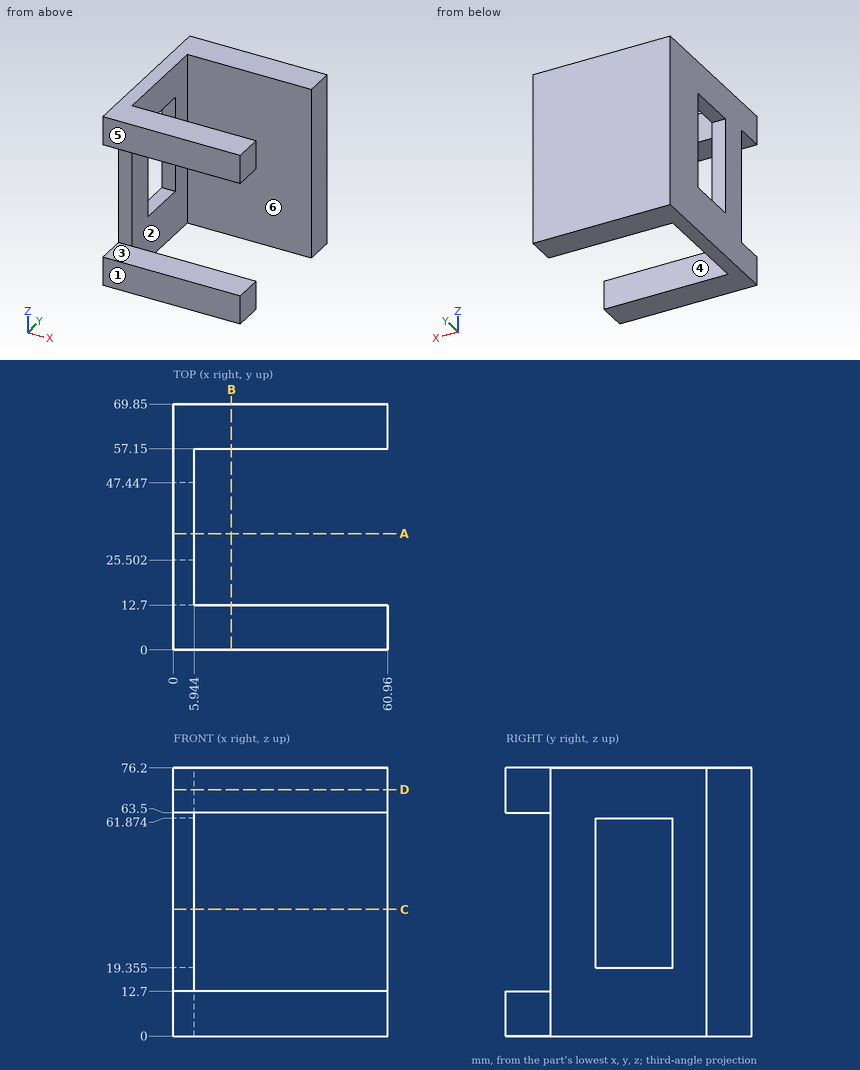
Geometry check sheet. Reference: drawing and pictorial views, mm from the part's lowest x, y, z. A direction names the side the tool comes from. Round coordinates to 2 decimals unless told otherwise and drop trailing zeros. Loops run counter-clockwise (first coordinate to the right, second up) from the corner with the lowest first, then second, coordinate; pieces in that order, holes last. Notation, with made-up numbers: (-7, 79) - (18, 79) arc R22 cw to (18, 92) - close; hole circle Ø8 at (-10.75, -30). An arc over 180 degrees is marked (long way). Use a Markdown table: item, result.
Q1. Draft check along Y on the marked faces 3, 4, 5 and 6. Enter one of: released by +Y, released by -Y, zero draft, split by the parting line, or undercut.
Solutions:
| item | result |
|---|---|
| face 3 | zero draft |
| face 4 | undercut |
| face 5 | released by -Y |
| face 6 | undercut |
Q2. Cross-section at B-B on x = 16.5. Record the cut outline in (y, z).
Solutions:
| item | result |
|---|---|
| outline | (0, 0) - (12.7, 0) - (12.7, 12.7) - (0, 12.7) - close; (0, 63.5) - (12.7, 63.5) - (12.7, 76.2) - (0, 76.2) - close; (57.15, 0) - (69.85, 0) - (69.85, 76.2) - (57.15, 76.2) - close |
Q3. Cross-section at C-C on z = 36. Record the cut outline in (x, y).
Solutions:
| item | result |
|---|---|
| outline | (0, 12.7) - (5.94, 12.7) - (5.94, 25.5) - (0, 25.5) - close; (0, 47.45) - (5.94, 47.45) - (5.94, 57.15) - (60.96, 57.15) - (60.96, 69.85) - (0, 69.85) - close |
Q4. Access from +Z, -Z, +X, -X, +Y, -Y to the whole of each face (thin tool, end or side, straight path). Record for the marked faces 1 and 2.
Solutions:
| item | result |
|---|---|
| face 1 | +Z, -Z, +X, -X, -Y |
| face 2 | +Z, -Z, +X |
Q5. Go/stop test with flat-tipped pins: P1, Ø5, axis at x = 3, z = 31, coming from the -Y side; P2, Ø10, axis at y = 19, z = 12.5, coming from the +X side; P3, Ø6.5, axis at x = 4.5, y = 36.5, coming from the -Z side. Record where each tip stops, or that it passes through.
Solutions:
| item | result |
|---|---|
| P1 | stops at y = 12.7 |
| P2 | stops at x = 5.94 |
| P3 | stops at z = 0 |
Q6. Cross-section at D-D on z = 70. Record the cut outline in (x, y), plus the area to 3 significant figures.
Solutions:
| item | result |
|---|---|
| outline | (0, 0) - (60.96, 0) - (60.96, 12.7) - (5.94, 12.7) - (5.94, 57.15) - (60.96, 57.15) - (60.96, 69.85) - (0, 69.85) - close |
| area | 1,810 mm2 |
Q7. Cross-section at A-A on y = 33. Record the cut outline in (x, z) (1 decimal).
Solutions:
| item | result |
|---|---|
| outline | (0, 0) - (5.9, 0) - (5.9, 19.4) - (0, 19.4) - close; (0, 61.9) - (5.9, 61.9) - (5.9, 76.2) - (0, 76.2) - close |
Q8. Material ranges on line 1 (Z direction, x = 36, y = 11.5); line 2 (Y direction, x = 46.5, z = 6); line 3 (Y direction, x = 43, z = 42.5), recorded low to high.
Solutions:
| item | result |
|---|---|
| line 1 | z = 0 to 12.7, 63.5 to 76.2 |
| line 2 | y = 0 to 12.7, 57.15 to 69.85 |
| line 3 | y = 57.15 to 69.85 |
